from build123d import *

# Parameters (mm, degrees)
F0_W     = 70
F0_H     = 160
F0_R     = 1.6
F0_R_2   = 1.75
F0_R_3   = 1.3
F0_R_4   = 13.65
F1_DEPTH = 2
F2_R     = 4


with BuildPart() as f1:
    # F0 (on Front) → F1 (new body)
    with BuildSketch(Plane.XZ):
        with Locations((0, -45)):
            Rectangle(F0_W, F0_H)
        with Locations((-26.851443, -117)):
            Circle(F0_R, mode=Mode.SUBTRACT)
        with Locations((-8.651443, -117)):
            Circle(F0_R, mode=Mode.SUBTRACT)
        with Locations((-26.851443, -76)):
            Circle(F0_R_2, mode=Mode.SUBTRACT)
        with Locations((-31.094084, -71.757359)):
            Circle(F0_R_3, mode=Mode.SUBTRACT)
        with Locations((-22.608802, -80.242641)):
            Circle(F0_R_3, mode=Mode.SUBTRACT)
        with Locations((-14.142136, -66.142136)):
            Circle(F0_R_2, mode=Mode.SUBTRACT)
        with Locations((9.548557, -117)):
            Circle(F0_R, mode=Mode.SUBTRACT)
        with Locations((27.748557, -117)):
            Circle(F0_R, mode=Mode.SUBTRACT)
        with Locations((14.142136, -66.142136)):
            Circle(F0_R_2, mode=Mode.SUBTRACT)
        with Locations((0, -52)):
            Circle(F0_R_4, mode=Mode.SUBTRACT)
        with Locations((22.608802, -80.242641)):
            Circle(F0_R_3, mode=Mode.SUBTRACT)
        with Locations((26.851443, -76)):
            Circle(F0_R_2, mode=Mode.SUBTRACT)
        with Locations((31.094084, -71.757359)):
            Circle(F0_R_3, mode=Mode.SUBTRACT)
        with Locations((-26.851443, -31.5)):
            Circle(F0_R_3, mode=Mode.SUBTRACT)
        with Locations((-26.851443, -25.5)):
            Circle(F0_R_2, mode=Mode.SUBTRACT)
        with Locations((-26.851443, -19.5)):
            Circle(F0_R_3, mode=Mode.SUBTRACT)
        with Locations((-14.142136, -37.857864)):
            Circle(F0_R_2, mode=Mode.SUBTRACT)
        with Locations((-14.142136, -14.142136)):
            Circle(F0_R_2, mode=Mode.SUBTRACT)
        with Locations((-31.437331, 22.982382)):
            Circle(F0_R_3, mode=Mode.SUBTRACT)
        with BuildLine():
            ThreePointArc((-25.101443, 26.851443), (-25.234654, 26.181747), (-25.614006, 25.614006))
            ThreePointArc((-25.614006, 25.614006), (-28.08888, 25.614006), (-28.08888, 28.08888))
            ThreePointArc((-28.08888, 28.08888), (-26.181747, 28.468232), (-25.101443, 26.851443))
        make_face(mode=Mode.SUBTRACT)
        with Locations((-22.265556, 30.720505)):
            Circle(F0_R_3, mode=Mode.SUBTRACT)
        with BuildLine():
            ThreePointArc((-12.392136, 14.142136), (-12.525346, 13.47244), (-12.904699, 12.904699))
            ThreePointArc((-12.904699, 12.904699), (-15.379572, 12.904699), (-15.379572, 15.379572))
            ThreePointArc((-15.379572, 15.379572), (-13.47244, 15.758925), (-12.392136, 14.142136))
        make_face(mode=Mode.SUBTRACT)
        with Locations((14.142136, -37.857864)):
            Circle(F0_R_2, mode=Mode.SUBTRACT)
        with Locations((14.142136, -14.142136)):
            Circle(F0_R_2, mode=Mode.SUBTRACT)
        with Locations((26.851443, -31.5)):
            Circle(F0_R_3, mode=Mode.SUBTRACT)
        with Locations((26.851443, -25.5)):
            Circle(F0_R_2, mode=Mode.SUBTRACT)
        with Locations((26.851443, -19.5)):
            Circle(F0_R_3, mode=Mode.SUBTRACT)
        with BuildLine():
            ThreePointArc((-9.652008, 9.652008), (5.223629, 12.610956), (13.65, 0))
            ThreePointArc((13.65, 0), (-5.223629, -12.610956), (-9.652008, 9.652008))
        make_face(mode=Mode.SUBTRACT)
        with Locations((14.142136, 14.142136)):
            Circle(F0_R_2, mode=Mode.SUBTRACT)
        with Locations((22.265556, 30.720505)):
            Circle(F0_R_3, mode=Mode.SUBTRACT)
        with Locations((31.437331, 22.982382)):
            Circle(F0_R_3, mode=Mode.SUBTRACT)
        with Locations((26.851443, 26.851443)):
            Circle(F0_R_2, mode=Mode.SUBTRACT)
    extrude(amount=F1_DEPTH)

    # F2
    f2_edges = [f1.edges().sort_by_distance(p)[0] for p in [
        (35, -1, 35),
        (35, -1, -125),
        (-35, -1, 35),
        (-35, -1, -125),
    ]]
    fillet(f2_edges, radius=F2_R)


solid = f1.part
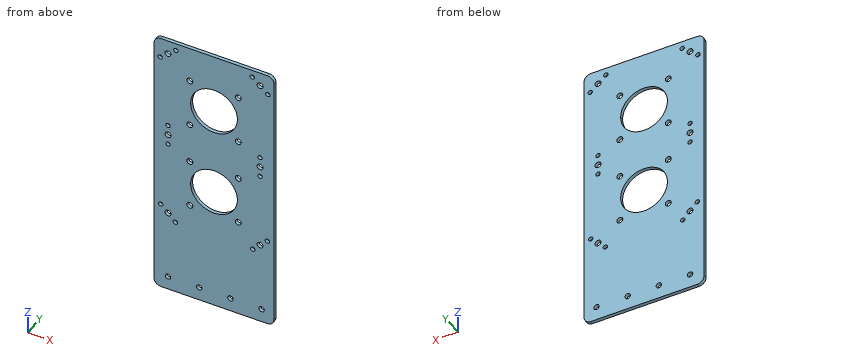
Design review of the part built by this model. Coordinates are the model's own, in mm. Give positions to 0.01 mm unless a question says otherwise; leave off trailing zeros. Write each loop counter-clockwise with the first axis right and the second up, starting at its lowest first coordinate (ties: lowest second). Pieces come first, ordered by that corner, then holes. Notation, with made-up numbers: M 57.25,-33.5 L 107.25,-33.5 A33 ccw 107.25,5.5 Z; hole C 16,53.5 d3. An arc over 180 degrees is marked long. Answer as a JSON object with one key per item and string values. Group by question number.
1) We need section C-C (z = -117). Give the boundary of the cut face in (x, y).
2) For line 1 along Z through (x, y) = (-0.5, -1.1); line 2 along Z through (x, y) = (-14, -1.7); line 3 along X through (y, z) = (-0.45, 24), list the stretches that pass through material, from the lowest coordinate up.
3) We need section B-B (x = 0). Give the boundary of the cut face in (y, z), and give its area (3 significant figures).
4) Clearance check with a flat-ended pin moving along its axis: pin 1 Ø2.5 at (x, z) = (-26.85, -19.5) entering from -Y. State where the tip first meets the part, or that it passes through.
5) We need section D-D (z = -25.5). Give the boundary of the cut face in (x, y).
6) We need section A-A (z = -52). Give the boundary of the cut face in (x, y).
Answer key:
{
 "1": {"outline": "M -35,-2 L -28.45,-2 L -28.45,0 L -35,0 Z; M -25.25,-2 L -10.25,-2 L -10.25,0 L -25.25,0 Z; M -7.05,-2 L 7.95,-2 L 7.95,0 L -7.05,0 Z; M 11.15,-2 L 26.15,-2 L 26.15,0 L 11.15,0 Z; M 29.35,-2 L 35,-2 L 35,0 L 29.35,0 Z"},
 "2": {"line 1": "z = -125 to -65.64, -38.36 to -13.64, 13.64 to 35", "line 2": "z = -125 to -67.89, -64.4 to -39.6, -36.11 to -15.89, -12.4 to 12.4, 15.89 to 35", "line 3": "x = -35 to -32.25, -30.63 to 30.63, 32.25 to 35"},
 "3": {"outline": "M -2,-125 L 0,-125 L 0,-65.65 L -2,-65.65 Z; M -2,-38.35 L 0,-38.35 L 0,-13.65 L -2,-13.65 Z; M -2,13.65 L 0,13.65 L 0,35 L -2,35 Z", "area": "211 mm²"},
 "4": {"pin 1": "passes through"},
 "5": {"outline": "M -35,-2 L -28.6,-2 L -28.6,0 L -35,0 Z; M -25.1,-2 L 25.1,-2 L 25.1,0 L -25.1,0 Z; M 28.6,-2 L 35,-2 L 35,0 L 28.6,0 Z"},
 "6": {"outline": "M -35,-2 L -13.65,-2 L -13.65,0 L -35,0 Z; M 13.65,-2 L 35,-2 L 35,0 L 13.65,0 Z"}
}
